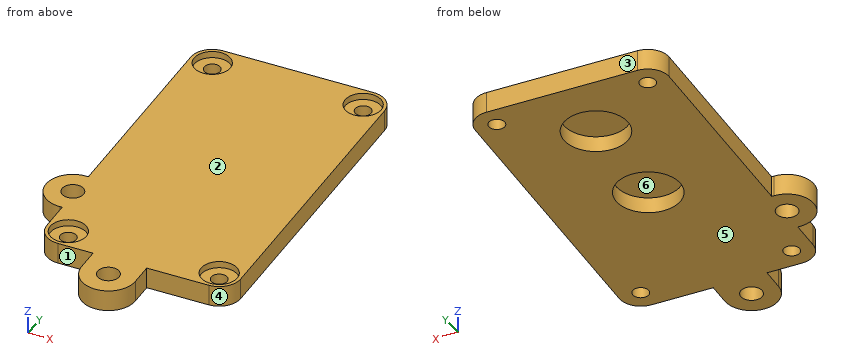
Autodesk Inventor part; units mm, degrees
ref_plane "YZ Plane" through (0, 0, 0) normal (1, 0, 0) x (0, 1, 0)
ref_plane "XZ Plane" through (0, 0, 0) normal (0, 1, 0) x (-1, 0, 0)
ref_plane "XY Plane" through (0, 0, 0) normal (0, 0, 1) x (1, 0, 0)
sketch "Эскиз1" plane through (0, 0, 0) normal (0, 0, 1) x (1, 0, 0)
  arc A0 (31.2016, -58.4471) -> (38.772, -50.0394) centre (30.783, -50.4581) ccw
  line L0 (31.2016, -58.4471) -> (8.1333, -59.6561)
  line L1 (33.0098, 59.9097) -> (38.772, -50.0394)
  arc A1 (33.0098, 59.9097) -> (24.6021, 67.4801) centre (25.0208, 59.491) ccw
  circle A2 centre (-2.0934, 39.9452) radius 12
  circle A3 centre (0, 0) radius 12
  line L2 (-34.9911, -22.1042) -> (-39.0912, 56.131)
  arc A4 (-35.8899, -22.1513) -> (-34.8432, -42.1239) centre (-35.3665, -32.1376) ccw
  line L3 (-34.9911, -22.1042) -> (-35.8899, -22.1513)
  line L4 (-34.8432, -42.1239) -> (-33.9444, -42.0768)
  line L5 (-33.3291, -53.8181) -> (-33.9444, -42.0768)
  arc A5 (-33.3291, -53.8181) -> (-24.9213, -61.3884) centre (-25.34, -53.3994) ccw
  line L6 (-11.8393, -60.7028) -> (-24.9213, -61.3884)
  arc A6 (-31.5209, 64.5388) -> (-39.0912, 56.131) centre (-31.1022, 56.5497) ccw
  line L7 (-31.5209, 64.5388) -> (24.6021, 67.4801)
  arc A7 (-11.3817, -69.4335) -> (8.5909, -68.3868) centre (-1.3954, -68.9101) ccw
  line L8 (-11.8393, -60.7028) -> (-11.3817, -69.4335)
  line L9 (8.5909, -68.3868) -> (8.1333, -59.6561)
  point P0 (24.6021, 67.4801)
  point P1 (26.2085, -58.7088)
extrude "Выдавливание1" add sketch "Эскиз1" along normal blind 6
sketch "Эскиз2" plane through (0, 0, 6) normal (0, 0, 1) x (1, 0, 0)
  line L0 (38.772, -50.0394) -> (33.0098, 59.9097)
  line L1 (8.1333, -59.6561) -> (31.2016, -58.4471)
  arc A0 (31.2016, -58.4471) -> (38.772, -50.0394) centre (30.783, -50.4581) ccw
  arc A1 (-33.3291, -53.8181) -> (-24.9213, -61.3884) centre (-25.34, -53.3994) ccw
  line L2 (-33.9444, -42.0768) -> (-33.3291, -53.8181)
  line L3 (-34.8432, -42.1239) -> (-33.9444, -42.0768)
  arc A2 (-35.8899, -22.1513) -> (-34.8432, -42.1239) centre (-35.3665, -32.1376) ccw
  line L4 (-39.0912, 56.131) -> (-34.9911, -22.1042)
  line L5 (-34.9911, -22.1042) -> (-35.8899, -22.1513)
  arc A3 (-31.5209, 64.5388) -> (-39.0912, 56.131) centre (-31.1022, 56.5497) ccw
  line L6 (24.6021, 67.4801) -> (-31.5209, 64.5388)
  arc A4 (33.0098, 59.9097) -> (24.6021, 67.4801) centre (25.0208, 59.491) ccw
  arc A5 (-11.3817, -69.4335) -> (8.5909, -68.3868) centre (-1.3954, -68.9101) ccw
  line L7 (-11.8393, -60.7028) -> (-11.3817, -69.4335)
  line L8 (-24.9213, -61.3884) -> (-11.8393, -60.7028)
  line L9 (8.5909, -68.3868) -> (8.1333, -59.6561)
  point P0 (0, 0)
extrude "Выдавливание2" add sketch "Эскиз2" along normal blind 2
sketch "Эскиз3" plane through (0, 0, 8) normal (0, 0, 1) x (1, 0, 0)
  circle A0 centre (25.0208, 59.491) radius 3 construction
  circle A1 centre (-31.1022, 56.5497) radius 3 construction
  circle A2 centre (30.783, -50.4581) radius 3 construction
  circle A3 centre (-25.34, -53.3994) radius 3 construction
  point P0 (0, 0)
hole "Отверстие1" at (-25.34, -53.3994, 8) at (30.783, -50.4581, 8) at (-31.1022, 56.5497, 8) at (25.0208, 59.491, 8) direction (0, 0, -1) diameter 6 end through all counterbore diameter 13.5 counterbore depth 2.5
sketch "Эскиз4" plane through (0, 0, 8) normal (0, 0, 1) x (1, 0, 0)
  circle A0 centre (-1.3954, -68.9101) radius 4 construction
  circle A1 centre (-35.3665, -32.1376) radius 4 construction
  point P0 (0, 0)
hole "Отверстие2" at (-1.3954, -68.9101, 8) at (-35.3665, -32.1376, 8) direction (0, 0, -1) diameter 8 end through all
properties part number "Пластина 2"
Can you work these out from the model? Positions are in its coordinate system, mm. Face numbers are marked on the shaded views. A direction names the side the tool comes from. Round coordinates to 2 decimals unless told otherwise and drop trailing zeros. Order: outer loops, then holes, each group sorted by start corner. A loop starts at its lowest first (then second) coordinate and runs counter-clockwise, first axis right, second up. Notation, with made-up numbers: (46.5, 66) -> (89.5, 66) arc R21 cw to (89.5, 82) -> close; hole circle Ø9 at (52.25, 75). An arc over 180 degrees is marked (long way). Return JSON: item names as keys, results as strings. Group by question number.
1. Will these pins go through, and if not, where does the flat tip stop? pin 1 (6.5 mm diameter, centred on x = -31.5, y = 59, fed in from +Z); pin 2 (21.5 mm diameter, centred on x = -2.09, y = 39.95, fed in from -Z); pin 3 (1 mm diameter, centred on x = 27.5, z = 2.5, fed in from -Y).
2. If we section it at C-C, the plane y = 0: Write out the boundary of the cut face in (x, z).
3. Which directions (+Z, -Z, +X, -X, +Y, -Y) give clear straight access to the entire face, cutting with the end or side of a thin tool? Please do the marked faces 5 and 6.
4. We'd pull the mould along X, two halves only. Please class the marked faces 1, 2, 3 and 4: released by +X, released by -X, zero draft, split by the parting line, or undercut.
5. If we section it at A-A, the plane x = 0: Write out the boundary of the cut face in (y, z), then the cut area to 3 significant figures.
6. If we section it at B-B, the plane z = 1.75: Count the separate pieces of the cut face and the enclosed holes in it, then the cut area to 3 significant figures.
7. I need wall thicknesses on line 1 (Z direction, x = 4, y = 4); line 2 (X direction, y = 30.5, z = 2.25); line 3 (X direction, y = 10, z = 0.5). Which ranges of each line are inside material? Lowest first, please. Write a range as [from, to].
Output values:
{
 "1": {"pin 1": "z = 5.5", "pin 2": "z = 6", "pin 3": "y = -58.67"},
 "2": {"outline": "(-36.15, 0) -> (-12, 0) -> (-12, 6) -> (12, 6) -> (12, 0) -> (36.15, 0) -> (36.15, 8) -> (-36.15, 8) -> close"},
 "3": {"face 5": "-Z, +X, -X, +Y, -Y", "face 6": "-Z"},
 "4": {"face 1": "undercut", "face 2": "zero draft", "face 3": "released by -X", "face 4": "released by +X"},
 "5": {"outline": "(-78.81, 0) -> (-72.66, 0) -> (-72.66, 8) -> (-78.81, 8) -> close; (-65.16, 0) -> (-12, 0) -> (-12, 6) -> (12, 6) -> (12, 0) -> (28.13, 0) -> (28.13, 6) -> (51.76, 6) -> (51.76, 0) -> (66.19, 0) -> (66.19, 8) -> (-65.16, 8) -> close", "area": "814 mm²"},
 "6": {"separate pieces": "1", "enclosed holes": "8", "area": "8,440 mm²"},
 "7": {"line 1": "[6, 8]", "line 2": "[-37.75, -9.5], [5.31, 34.55]", "line 3": "[-36.67, -6.63], [6.63, 35.63]"}
}
